Can you work these out from the model? Positions are in its coordinate system, mm. A direction names the side the tool comes from. Coordinates: 2 decimals unless noted, no trailing zeros. Order: outer loops, then holes, each group sorted by start corner. A loop starts at its lowest first (then second) coordinate and runs counter-clockwise, first axis right, second up. Notation, with made-up numbers: (83.5, 51.5) - (129.5, 51.5) arc R17 cw to (129.5, 71.5) - close; hole circle Ø10 at (1.5, 85). An arc over 180 degrees is marked (long way). Use a Markdown table: item, result. Add a question column.
(1) I want a section at A-A (x = 0). List the corners of the cut face in (y, z) for me, and give its area (3 significant figures).
(2) On a 3-axis mill with a long thin cutter (end or side, diameter ignored), from which of +Z, -Z, +X, -X, +Y, -Y can I reach the whole of each face in a straight line? I mean faces 1 (the cylindrical face through (24.327, -30.148, 22.398)), 2 (the flat face through (11, -44.571, 21)). Say none if no direction works.
(3) For pin 1 Ø3 at (y, z) = (-25.5, 30) entering from +X; pin 2 Ø8 at (x, z) = (-30.5, 53) entering from -Y; pin 3 Ø1 at (x, y) = (43, 3.5) entering from -Z, each with a flat end and sliding along its axis, tell me the tip position at first contact or that it passes through.
(4) I want a section at B-B (z = 9). List the corners of the cut face in (x, y) for me.
(5) I want a section at C-C (y = -30). List the corners of the cut face in (x, z) for me, and give its area (3 significant figures).
(6) If I drill on L1, parallel to Z at x = 0, y = -25.75; L2, parallel to Z at x = 0, y = -1; L3, parallel to Y at x = 31.5, z = 5, over which ranges is the centre line in solid material (lowest first)? Write a range as [from, to].
(7) I want a section at D-D (x = -13). List the corners of the cut face in (y, z) for me, and give its area (3 significant figures).
```python
from build123d import *

# Parameters (mm, degrees)
F0_W     = 118.841722
F0_H     = 32.246224
F1_DEPTH = 69.088
F2_R     = 15.064015
F3_DEPTH = 104.648
F2_R_2   = 26.33517
F4_DEPTH = 28.448


with BuildPart() as f1:
    # F0 (on Top) → F1 (new body)
    with BuildSketch(Plane.XY):
        Rectangle(F0_W, F0_H)
    extrude(amount=F1_DEPTH)

    # F2 (on face) → F3 (cut)
    with BuildSketch(Plane.XZ.offset(16.123112)):
        with Locations((0, 32.48496)):
            Circle(F2_R)
    extrude(amount=-F3_DEPTH, mode=Mode.SUBTRACT)

    # F2 (on face) → F4 (join)
    with BuildSketch(Plane.XZ.offset(16.123112)):
        with Locations((0, 32.48496)):
            Circle(F2_R_2)
        with Locations((0, 32.48496)):
            Circle(F2_R, mode=Mode.SUBTRACT)
    extrude(amount=F4_DEPTH)


solid = f1.part
```
Answers follow:
| question | item | result |
|---|---|---|
| 1 | outline | (-44.57, 6.15) - (-16.12, 6.15) - (-16.12, 0) - (16.12, 0) - (16.12, 17.42) - (-44.57, 17.42) - close; (-44.57, 47.55) - (16.12, 47.55) - (16.12, 69.09) - (-16.12, 69.09) - (-16.12, 58.82) - (-44.57, 58.82) - close |
| 1 | area | 1,900 mm² |
| 2 | face 1 | -Y |
| 2 | face 2 | +Z, -Z, +X, -X, -Y |
| 3 | pin 1 | stops at x = 26.32 |
| 3 | pin 2 | stops at y = -16.12 |
| 3 | pin 3 | stops at z = 0 |
| 4 | outline | (-59.42, -16.12) - (-11.92, -16.12) - (-11.92, -44.57) - (11.92, -44.57) - (11.92, -16.12) - (59.42, -16.12) - (59.42, 16.12) - (-59.42, 16.12) - close |
| 5 | outline | circle Ø52.67 at (0, 32.48); hole circle Ø30.13 at (0, 32.48) |
| 5 | area | 1,470 mm² |
| 6 | L1 | z = [6.15, 17.42], [47.55, 58.82] |
| 6 | L2 | z = [0, 17.42], [47.55, 69.09] |
| 6 | L3 | y = [-16.12, 16.12] |
| 7 | outline | (-44.57, 9.58) - (-16.12, 9.58) - (-16.12, 0) - (16.12, 0) - (16.12, 24.87) - (-44.57, 24.87) - close; (-44.57, 40.1) - (16.12, 40.1) - (16.12, 69.09) - (-16.12, 69.09) - (-16.12, 55.39) - (-44.57, 55.39) - close |
| 7 | area | 2,610 mm² |
